Read the model definition and answer for the solid it produces. Units are mm, in the model's axes. Face numbers are marked on the shaded views. A direction names the side the tool comes from. Give positions to 0.01 mm unless a question says otherwise; leave off trailing zeros. Order: outer loops, then holes, each group sorted by start corner. A loop starts at its lowest first (then second) coordinate and runs counter-clockwise, first axis right, second up. Notation, with made-up numbers: (62, -39.75) - (106, -39.75) arc R17 cw to (106, -8.75) - close; hole circle Ø5 at (37, 20). An arc over 180 degrees is marked (long way). Return JSON: item names as keys, results as strings.
```python
from build123d import *

# Parameters (mm, degrees)
SKETCH1_W                                      = 60
SKETCH1_H                                      = 60
EXTRUDE1_DEPTH                                 = 10
SKETCH3_R                                      = 5
EXTRUDE2_DEPTH                                 = 44.588989435
SKETCH5_R                                      = 19.05
EXTRUDE3_DEPTH                                 = 1.5
SKETCH6_R                                      = 22.4
EXTRUDE4_DEPTH                                 = 4
SKETCH7_R                                      = 2.25
EXTRUDE6_DEPTH                                 = 44.588989435
SKETCH8_R                                      = 2.25
EXTRUDE7_DEPTH                                 = 44.269504273
CSK_FOR_M4_FLAT_HEAD_MACHINE_SCREW1_AT_2_COUNT = 2
CSK_FOR_M4_FLAT_HEAD_MACHINE_SCREW1_AT_2_PITCH = 21.213203436
CSK_FOR_M4_FLAT_HEAD_MACHINE_SCREW1_AT_3_COUNT = 2
CSK_FOR_M4_FLAT_HEAD_MACHINE_SCREW1_AT_3_PITCH = 30
CSK_FOR_M4_FLAT_HEAD_MACHINE_SCREW1_AT_4_COUNT = 2
CSK_FOR_M4_FLAT_HEAD_MACHINE_SCREW1_AT_4_PITCH = 21.213203436


with BuildPart() as part:
    # Sketch1 → Extrude1 (new body)
    with BuildSketch(Plane(origin=(0, 0, 0), x_dir=(0, 0, -1), z_dir=(1, 0, 0))):
        Rectangle(SKETCH1_W, SKETCH1_H)
    extrude(amount=EXTRUDE1_DEPTH)

    # Sketch3 → Extrude2 (cut, through all)
    with BuildSketch(Plane(origin=(10, 0, 0), x_dir=(0, 0, -1), z_dir=(1, 0, 0))):
        Circle(SKETCH3_R)
    extrude(amount=-EXTRUDE2_DEPTH, mode=Mode.SUBTRACT)

    # Sketch5 → Extrude3 (cut)
    with BuildSketch(Plane(origin=(10, 0, 0), x_dir=(0, 0, -1), z_dir=(1, 0, 0))):
        Circle(SKETCH5_R)
    extrude(amount=-EXTRUDE3_DEPTH, mode=Mode.SUBTRACT)

    # Sketch6 → Extrude4 (cut)
    with BuildSketch(Plane.ZY):
        Circle(SKETCH6_R)
    extrude(amount=-EXTRUDE4_DEPTH, mode=Mode.SUBTRACT)

    # Sketch7 → Extrude6 (cut, through all)
    with BuildSketch(Plane.ZY):
        with Locations((23.57, 23.57)):
            Circle(SKETCH7_R)
        with Locations((-23.57, 23.57)):
            Circle(SKETCH7_R)
        with Locations((23.57, -23.57)):
            Circle(SKETCH7_R)
        with Locations((-23.57, -23.57)):
            Circle(SKETCH7_R)
    extrude(amount=-EXTRUDE6_DEPTH, mode=Mode.SUBTRACT)

    # Sketch8 → Extrude7 (cut, through all)
    with BuildSketch(Plane(origin=(8.5, 0, 0), x_dir=(0, 0, -1), z_dir=(1, 0, 0))):
        with Locations((0, 15)):
            Circle(SKETCH8_R)
        with Locations((-15, 0)):
            Circle(SKETCH8_R)
        with Locations((0, -15)):
            Circle(SKETCH8_R)
        with Locations((15, 0)):
            Circle(SKETCH8_R)
    extrude(amount=-EXTRUDE7_DEPTH, mode=Mode.SUBTRACT)

    # Sketch9 → CSK for M4 Flat Head Machine Screw1 (revolve, cut)
    with BuildSketch(Plane(origin=(8.5, 15, 0), x_dir=(0, 0, -1), z_dir=(0, 1, 0))):
        Polygon((0, 0), (0, 8.5), (2.25, 8.5), (2.25, 2.45), (4.7, 0), align=None)
    csk_for_m4_flat_head_machine_screw1 = revolve(axis=Axis((14.85, 15, 0), (-1, 0, 0)), mode=Mode.SUBTRACT)

    # CSK for M4 Flat Head Machine Screw1 at 2: CSK for M4 Flat Head Machine Screw1 ×2
    with Locations(*[Vector(0, -0.7071067811865476, 0.7071067811865476) * (i * CSK_FOR_M4_FLAT_HEAD_MACHINE_SCREW1_AT_2_PITCH) for i in range(1, CSK_FOR_M4_FLAT_HEAD_MACHINE_SCREW1_AT_2_COUNT)]):
        add(csk_for_m4_flat_head_machine_screw1, mode=Mode.SUBTRACT)

    # CSK for M4 Flat Head Machine Screw1 at 3: CSK for M4 Flat Head Machine Screw1 ×2
    with Locations(*[(0, -i * CSK_FOR_M4_FLAT_HEAD_MACHINE_SCREW1_AT_3_PITCH, 0) for i in range(1, CSK_FOR_M4_FLAT_HEAD_MACHINE_SCREW1_AT_3_COUNT)]):
        add(csk_for_m4_flat_head_machine_screw1, mode=Mode.SUBTRACT)

    # CSK for M4 Flat Head Machine Screw1 at 4: CSK for M4 Flat Head Machine Screw1 ×2
    with Locations(*[Vector(0, -0.7071067811865476, -0.7071067811865476) * (i * CSK_FOR_M4_FLAT_HEAD_MACHINE_SCREW1_AT_4_PITCH) for i in range(1, CSK_FOR_M4_FLAT_HEAD_MACHINE_SCREW1_AT_4_COUNT)]):
        add(csk_for_m4_flat_head_machine_screw1, mode=Mode.SUBTRACT)


solid = part.part
```
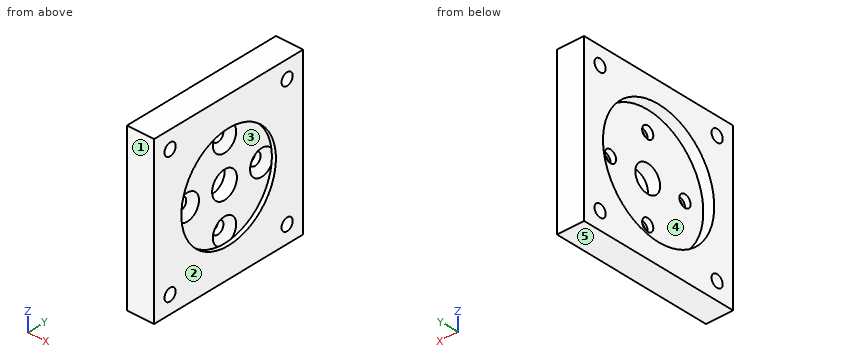
Q1. A cutting plane is placed at B-B (z = 23.57). Write down the section's boundary in (x, y).
Values:
{"outline": "(0, -30) - (10, -30) - (10, -25.82) - (0, -25.82) - close; (0, -21.32) - (10, -21.32) - (10, 21.32) - (0, 21.32) - close; (0, 25.82) - (10, 25.82) - (10, 30) - (0, 30) - close"}
Q2. Given pin 1 (6 mm diameter, centred on y = -23.57, z = 23.57, fed in from -X); pin 2 (0.7 mm diameter, centred on y = 19.5, z = -1, fed in from -X); pin 3 (11.5 mm diameter, centred on y = 3, z = 1, fed in from +X); pin 4 (4 mm diameter, centred on y = 23.57, z = -23.57, fed in from +X), each flat-ended and moving along its own axis, determine where each tip first touches the part or whether it passes through.
Values:
{"pin 1": "stops at x = 0", "pin 2": "stops at x = 4", "pin 3": "stops at x = 8.5", "pin 4": "passes through"}
Q3. Determine the mould class of the marked faces 1, 2 and 3 for opening direction Y: released by +Y, released by -Y, zero draft, split by the parting line, or undercut.
Values:
{"face 1": "released by -Y", "face 2": "zero draft", "face 3": "undercut"}
Q4. For the marked faces 4 and 5, determine the directions among +Z, -Z, +X, -X, +Y, -Y from which every point of the face is accessible in a straight line to the end or side of a thin tool.
Values:
{"face 4": "-X", "face 5": "-Z, +X, -X, +Y, -Y"}
Q5. A cutting plane is placed at D-D (x = 7.25). Give the number of separate pieces and of enclosed holes in the cut face, and give its area (3 significant figures).
Values:
{"separate pieces": "1", "enclosed holes": "9", "area": "3,310 mm²"}
Q6. A cutting plane is placed at C-C (y = -15). Write down the section's boundary in (x, z), and give its area (3 significant figures).
Values:
{"outline": "(0, -30) - (10, -30) - (10, -11.74) - (8.5, -11.74) - (8.5, -4.7) - (6.05, -2.25) - (4, -2.25) - (4, -16.64) - (0, -16.64) - close; (0, 16.64) - (4, 16.64) - (4, 2.25) - (6.05, 2.25) - (8.5, 4.7) - (8.5, 11.74) - (10, 11.74) - (10, 30) - (0, 30) - close", "area": "405 mm²"}
Q7. A cutting plane is placed at A-A (x = 3). Write down the section's boundary in (y, z).
Values:
{"outline": "(-30, -30) - (30, -30) - (30, 30) - (-30, 30) - close; hole circle Ø4.5 at (-23.57, -23.57); hole circle Ø4.5 at (-23.57, 23.57); hole circle Ø44.8 at (0, 0); hole circle Ø4.5 at (23.57, -23.57); hole circle Ø4.5 at (23.57, 23.57)"}
Q8. Consider L1, parallel to Y at x = 4.55, z = 0; L2, parallel to Z at x = 3.75, y = 0.5; L3, parallel to Y at x = 5.05, z = -15. Determine where each line is inside the solid, lowest interval first.
Values:
{"L1": "y = -30 to -17.25, -12.75 to -5, 5 to 12.75, 17.25 to 30", "L2": "z = -30 to -22.39, 22.39 to 30", "L3": "y = -30 to -2.25, 2.25 to 30"}
